Can you work these out from the model? Positions are in its coordinate system, mm. A direction names the side the tool comes from. Round coordinates to 2 decimals unless told otherwise and drop trailing zeros. Loops run counter-clockwise (first coordinate to the right, second up) from the corner with the lowest first, then second, coordinate; pieces in that order, holes last. Notation, with made-up numbers: M -32,78 L -23,78 A19 cw -23,97 Z; hole C -27.75,-35.5 d2. An arc over 180 degrees is marked long. Return JSON: item names as keys, results as strings.
```python
from build123d import *

# Parameters (mm, degrees)
SKETCH_1_W          = 9.1
SKETCH_1_H          = 4
EXTRUDE_1_DEPTH     = 10
SKETCH_2_R          = 0.5
SKETCH_2_R_2        = 1
CUT_EXTRUDE_1_DEPTH = 14.667845478
SKETCH_3_R          = 0.8
CUT_EXTRUDE_2_DEPTH = 2


with BuildPart() as part:
    # Sketch 1 → Extrude 1 (new body)
    with BuildSketch(Plane(origin=(0, 0, 0), x_dir=(1, 0, 0), z_dir=(0, 1, 0))):
        Rectangle(SKETCH_1_W, SKETCH_1_H)
    extrude(amount=EXTRUDE_1_DEPTH)

    # Sketch 2 → Cut-Extrude 1 (cut, through all)
    with BuildSketch(Plane.ZY.offset(4.55)):
        with Locations((0, 7)):
            Circle(SKETCH_2_R)
        with Locations((2.1, 2)):
            Circle(SKETCH_2_R_2)
    extrude(amount=-CUT_EXTRUDE_1_DEPTH, mode=Mode.SUBTRACT)

    # Sketch 3 → Cut-Extrude 2 (cut)
    with BuildSketch(Plane(origin=(0, 10, 0), x_dir=(1, 0, 0), z_dir=(0, 1, 0))):
        with Locations(Location((3.05, 0, 0), (0, 0, 270))):
            Circle(SKETCH_3_R)
        with Locations(Location((-3.05, 0, 0), (0, 0, 270))):
            Circle(SKETCH_3_R)
    extrude(amount=-CUT_EXTRUDE_2_DEPTH, mode=Mode.SUBTRACT)


solid = part.part
```
Q1. On a 3-axis mill with a long thin cutter (end or side, diameter ignored), from which of +Z, -Z, +X, -X, +Y, -Y can I reach the whole of each face in a straight line? I mean faces 4 (the flat face through (0, 5, -2)), 5 (the cylindrical face through (2.27, 9.01, -0.17)). Say none if no direction works.
Results:
{"face 4": "-Z, +X, -X, +Y, -Y", "face 5": "+Y"}
Q2. If I drill on line 1 along X through (y, z) = (9.05, 0); line 2 along Y through (x, z) = (-1, 0); line 3 along Z through (x, y) = (-2, 2), over which ranges is the centre line in solid material (lowest first)?
Results:
{"line 1": "x = -4.55 to -3.85, -2.25 to 2.25, 3.85 to 4.55", "line 2": "y = 0 to 6.5, 7.5 to 10", "line 3": "z = -2 to 1.1"}
Q3. Suppose I cut it at B-B, the plane x = 1. Please give me the cut outline in (y, z).
Results:
{"outline": "M 0,-2 L 10,-2 L 10,2 L 2.99,2 A1 cw 1.01,2 L 0,2 Z; hole C 7,0 d1"}
Q4. Thinking about a two-plate mould opening in X: for faces 1 (the flat face through (4.55, 5, 0)), 2 (the flat face through (0, 6, 2)), 3 (the flat face through (3, 8, 0)), which applies, pulls with the +X half, pulls with the -X half, needs draft (parallel to the pull), parting line crosses it, or undercut?
Results:
{"face 1": "pulls with the +X half", "face 2": "needs draft", "face 3": "undercut"}
Q5. Suppose I cut it at C-C, the plane y = 7. Please give me the cut outline in (x, z), plus the area to 3 significant figures.
Results:
{"outline": "M -4.55,-2 L 4.55,-2 L 4.55,-0.5 L -4.55,-0.5 Z; M -4.55,0.5 L 4.55,0.5 L 4.55,2 L -4.55,2 Z", "area": "27.3 mm2"}
Q6. Suppose I cut it at A-A, the plane z = 0. Please give me the cut outline in (x, y), plus the area to 3 significant figures.
Results:
{"outline": "M -4.55,0 L 4.55,0 L 4.55,6.5 L -4.55,6.5 Z; M -4.55,7.5 L 4.55,7.5 L 4.55,10 L 3.85,10 L 3.85,8 L 2.25,8 L 2.25,10 L -2.25,10 L -2.25,8 L -3.85,8 L -3.85,10 L -4.55,10 Z", "area": "75.5 mm2"}
Q7. Suppose I cut it at D-D, the plane y = 8.5. Please give me the cut outline in (x, z).
Results:
{"outline": "M -4.55,-2 L 4.55,-2 L 4.55,2 L -4.55,2 Z; hole C -3.05,0 d1.6; hole C 3.05,0 d1.6"}
